Autodesk Inventor part; units mm, degrees
ref_plane "Start Plane" through (0, 0, 0) normal (0, 0, 1) x (1, 0, 0)
ref_plane "End Plane" through (0, 0, 440.875) normal (0, 0, 1) x (1, 0, 0)
ref_plane "Work Plane4" through (15.875, 0, 440.875) normal (-0.7071, 0, 0.7071) x (0.7071, 0, 0.7071)
ref_plane "Start Plane" through (0, 0, 0) normal (0, 0, 1) x (1, 0, 0)
ref_plane "End Plane" through (0, 0, 440.875) normal (0, 0, 1) x (1, 0, 0)
sketch "Sketch" plane through (0, 0, 0) normal (0, 0, 1) x (1, 0, 0)
  line L0 (-15.875, -9.525) -> (-15.875, 9.525)
  line L1 (-9.525, 15.875) -> (9.525, 15.875)
  line L2 (15.875, 9.525) -> (15.875, -9.525)
  line L3 (9.525, -15.875) -> (-9.525, -15.875)
  arc A0 (-15.875, -9.525) -> (-9.525, -15.875) centre (-9.525, -9.525) ccw
  arc A1 (-9.525, 15.875) -> (-15.875, 9.525) centre (-9.525, 9.525) ccw
  arc A2 (15.875, 9.525) -> (9.525, 15.875) centre (9.525, 9.525) ccw
  arc A3 (9.525, -15.875) -> (15.875, -9.525) centre (9.525, -9.525) ccw
  arc A4 (-9.525, 12.7) -> (-12.7, 9.525) centre (-9.525, 9.525) ccw
  line L4 (-9.525, 12.7) -> (9.525, 12.7)
  arc A5 (12.7, 9.525) -> (9.525, 12.7) centre (9.525, 9.525) ccw
  line L5 (12.7, 9.525) -> (12.7, -9.525)
  arc A6 (9.525, -12.7) -> (12.7, -9.525) centre (9.525, -9.525) ccw
  line L6 (9.525, -12.7) -> (-9.525, -12.7)
  arc A7 (-12.7, -9.525) -> (-9.525, -12.7) centre (-9.525, -9.525) ccw
  line L7 (-12.7, -9.525) -> (-12.7, 9.525)
  line L8 (0, 24.0662) -> (0, -24.0662) construction
  line L9 (-24.0662, 0) -> (24.0662, 0) construction
  dimension "d10" = 31.75
  dimension "d11" = 31.75
  dimension "d12" = 3.175
  dimension "d15" = 15.875
  dimension "d16" = 15.875
  dimension "d17" = 6.35
extrude "Body" add sketch "Sketch" along normal up to surface (440.875 mm away) from surface at 0
sketch "Sketch3" plane through (0, 0, 0) normal (0, 0, 1) x (1, 0, 0)
  line L0 (0, 0) -> (10, 0)
ref_plane "Work Plane3" through (0, 0, 0) normal (0, -1, 0) x (1, 0, 0)
sketch "Sketch4" plane through (0, 0, 0) normal (0, -1, 0) x (1, 0, 0)
  line L0 (-2, 0) -> (12, 0)
  line L1 (-2, 440.875) -> (12, 440.875)
  dimension "d19" = 440.875
ref_plane "Work Plane4" through (15.875, 0, 440.875) normal (-0.7071, 0, 0.7071) x (0.7071, 0, 0.7071)
split "Split1" plane through (15.875, 0, 440.875) removes the side toward (-0.7071, 0, 0.7071)
equation "\"d10\" = G_H"
equation "\"d11\" = G_W"
equation "\"d12\" = G_T"
equation "\"d15\" = 0.5 * d10"
equation "\"d16\" = 0.5 * d11"
equation "\"d17\" = G_IR"
equation "\"d3\" = G_L"
equation "\"G_W\" = 31.75"
equation "\"G_H\" = 31.75"
equation "\"G_T\" = 3.175"
equation "\"G_IR\" = 6.35"
equation "\"G_L\" = d19"
equation "\"G_OFFSET_START\" = 0"
equation "\"G_OFFSET_END\" = 15.875"
equation "\"d14\" = G_OFFSET_END + B_L"
equation "\"B_L\" = 425"
properties part number "AISC HSS - (1 1/4x1 1/4x1/8) - 17.357" material "Steel, Mild"
Geometry check sheet. Reference: the model listing, model coordinates, mm. A direction names the side the tool comes from. Round coordinates to 2 decimals unless told otherwise and drop trailing zeros. Order: outer loops, then holes, each group sorted by start corner. A loop starts at its lowest first (then second) coordinate and runs counter-clockwise, first axis right, second up. Notation, with made-up numbers: M 34,47.25 L 54,47.25 A29 ccw 54,81.25 Z; hole C 53.25,10 d5. An arc over 180 degrees is marked long. Write item = value, one per line.
Q1. Section check B-B (y = 2.5). Enter the section's corners in (x, z) (3 decimals).
Answer block:
outline = M -15.875,0 L -12.7,0 L -12.7,412.3 L -15.875,409.125 Z; M 12.7,0 L 15.875,0 L 15.875,440.875 L 12.7,437.7 Z
Q2. Release check for a two-part mould opening along X. For faces 1 (the flat face through (0, -12.7, 214)), 2 (the flat face through (-13, 0, 0)), 3 (the flat face through (15.875, 0, 217)), 4 (the flat face through (0, -13, 425)) record: released by +X, released by -X, zero draft, split by the parting line, or undercut.
Answer block:
face_1 = undercut
face_2 = zero draft
face_3 = released by +X
face_4 = released by -X
Q3. Section check C-C (z = 163). Enter the section's corners in (x, y) (3 decimals).
Answer block:
outline = M -15.875,-9.525 A6.35 ccw -9.525,-15.875 L 9.525,-15.875 A6.35 ccw 15.875,-9.525 L 15.875,9.525 A6.35 ccw 9.525,15.875 L -9.525,15.875 A6.35 ccw -15.875,9.525 Z; hole M -12.7,-9.525 A3.175 ccw -9.525,-12.7 L 9.525,-12.7 A3.175 ccw 12.7,-9.525 L 12.7,9.525 A3.175 ccw 9.525,12.7 L -9.525,12.7 A3.175 ccw -12.7,9.525 Z
Q4. Scan lines: line 1 (X direction, y = -7, z = 240) (3 decimals); line 2 (X direction, y = -11.5, z = 309.5). Record each from-to range of solid material in increasing order.
Answer block:
line_1 = -15.875 to -12.7, 12.7 to 15.875
line_2 = -15.56 to -12.01, 12.01 to 15.56
Q5. Section check A-A (x = 5). Enter the section's corners in (y, z) (3 decimals).
Answer block:
outline = M -15.875,0 L -12.7,0 L -12.7,430 L -15.875,430 Z; M 12.7,0 L 15.875,0 L 15.875,430 L 12.7,430 Z
Q6. Depth check by flat-ended pin: pin 1 Ø4 at (y, z) = (-10.5, 223.5) entering from +X (3 decimals); pin 2 Ø6 at (x, y) = (-2, 12.5) entering from +Z; pin 3 Ø2 at (x, z) = (-12.5, 299) entering from -Y; pin 4 Ø1.5 at (y, z) = (11.5, 200.5) entering from +X. Enter the tip coordinate at first touch or a pass-through.
Answer block:
pin_1 = 15.875
pin_2 = 425.99
pin_3 = -15.56
pin_4 = 15.76
Q7. Set-up check for faces 5 (the flat face through (0, 15.875, 214)), 6 (the flat face through (-12.7, 0, 203)): record each of +Z, -Z, +X, -X, +Y, -Y from which the full face is reachable in a straight line by a thin tool's end or side.
Answer block:
face_5 = +Z, -Z, +X, -X, +Y
face_6 = +Z, -Z
